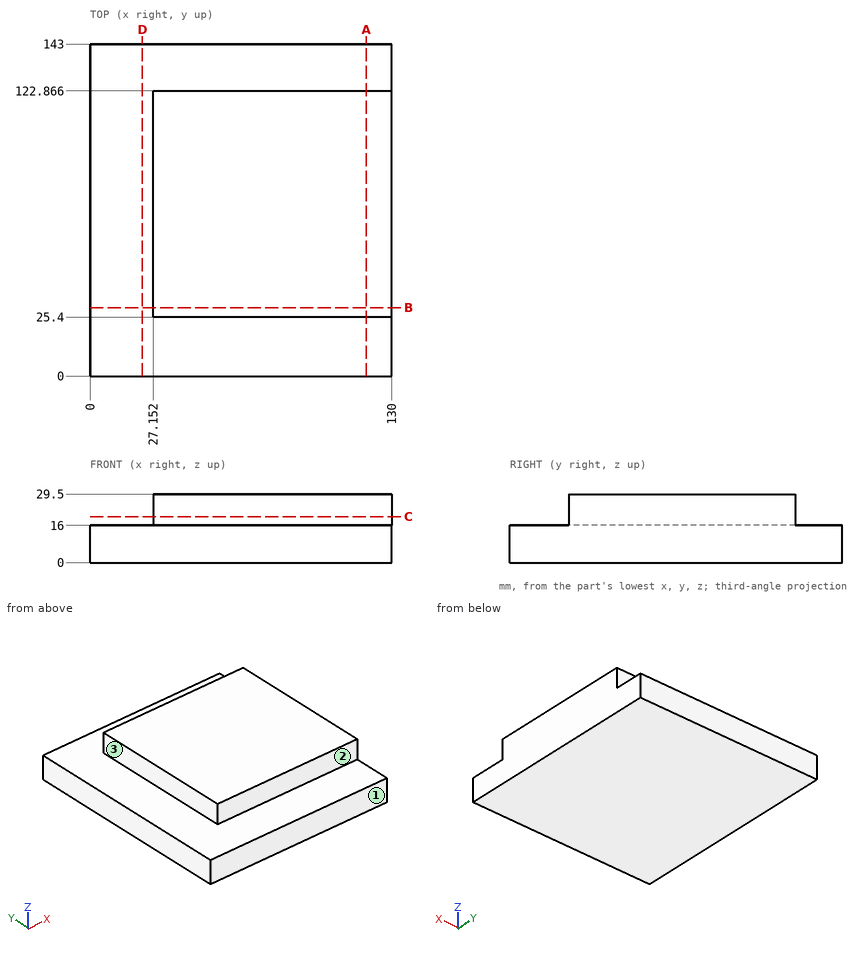
The figure shows three views and two pictorial views of one solid part (mm, origin at its lowest corner). Answer the questions. A direction names the side the tool comes from. Give positions to 0.01 mm unless a question says otherwise; leave off trailing zeros. Write each loop counter-clockwise with the first axis right and the second up, starting at its lowest first coordinate (ties: lowest second). Pieces come first, ordered by that corner, then holes. Notation, with made-up numbers: M 80,87.5 L 90,87.5 A8 ccw 90,102.5 Z; hole C 59,50 d7. An arc over 180 degrees is marked long. One line per item, written item: value. Start each with the question number.
(1) Find section D-D (x = 22.5). Determine the outline of the cut face in (y, z).
(2) Find section C-C (z = 19.75). Determine the outline of the cut face in (x, y).
(3) Find section B-B (y = 29.5). Determine the outline of the cut face in (x, z), plus the area to 3 significant figures.
(4) Find section A-A (x = 119). Determine the outline of the cut face in (y, z), plus the area to 3 significant figures.
(5) A tool of negligible diameter and unlimited length cuts with its end or side. For the marked faces 1, 2 and 3, from which of +Z, -Z, +X, -X, +Y, -Y can it reach the whole face along a straight path? Write none if from no direction.
(6) Find the intervals of material crossed by line 1 (Z direction, x = 50, y = 137); line 2 (X direction, y = 104.5, z = 20.75); line 3 (Y direction, x = 58, z = 21.5), in increasing order.
(7) Flat-ended cylindrical pins translate along their axes: pin 1 Ø4 at (x, z) = (100.5, 20) entering from -Y; pin 2 Ø10 at (y, z) = (54, 24.5) entering from -X. Find the tip coordinate at first contact, or state that the pin passes through.
Results below:
1. outline: M 0,0 L 143,0 L 143,16 L 0,16 Z
2. outline: M 27.15,25.4 L 130,25.4 L 130,122.87 L 27.15,122.87 Z
3. outline: M 0,0 L 130,0 L 130,29.5 L 27.15,29.5 L 27.15,16 L 0,16 Z
3. area: 3,470 mm^2
4. outline: M 0,0 L 143,0 L 143,16 L 122.87,16 L 122.87,29.5 L 25.4,29.5 L 25.4,16 L 0,16 Z
4. area: 3,600 mm^2
5. face 1: +Z, -Z, +X, -X, -Y
5. face 2: +Z, +X, -X, -Y
5. face 3: +Z, -X, +Y, -Y
6. line 1: z = 0 to 16
6. line 2: x = 27.15 to 130
6. line 3: y = 25.4 to 122.87
7. pin 1: stops at y = 25.4
7. pin 2: stops at x = 27.15
